Source: CAD feature listing. Evaluate the final solid. Frame: model axes, mm. Face numbers are marked on the shaded views. A direction names the side the tool comes from. Coordinates: 2 decimals unless noted, no trailing zeros. Loops run counter-clockwise (first coordinate to the right, second up) from the corner with the lowest first, then second, coordinate; pieces in that order, holes last. Notation, with made-up numbers: (53, -36) -> (61, -36) arc R35 cw to (61, 2) -> close; hole circle Ø1 at (15, 4). An arc over 180 degrees is marked (long way). Answer as CSV lines item,"result".
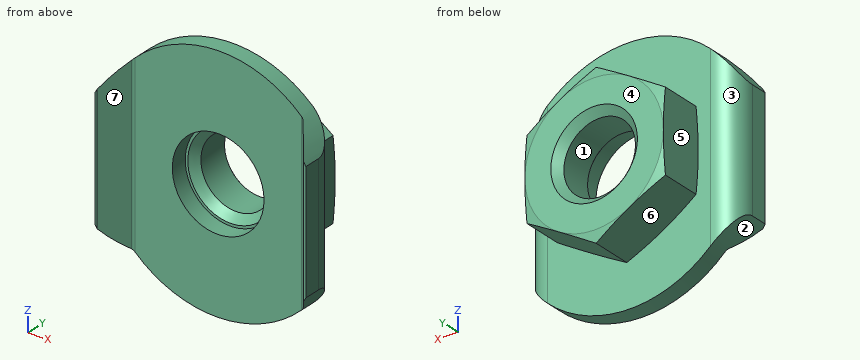
Autodesk Inventor part; units mm, degrees
ref_plane "FS1_XY" through (0, 0, 0) normal (0, 1, 0) x (1, 0, 0)
ref_plane "FS1_YZ" through (0, 0, 0) normal (1, 0, 0) x (0, 0, -1)
ref_plane "FS1_ZX" through (0, 0, 0) normal (0, 0, -1) x (0, 1, 0)
sketch "Skizze_1" plane through (0, 0, 0) normal (0, 0, 1) x (1, 0, 0)
  line L0 (-6.094, 2.6187) -> (-5.9701, 2.6187)
  line L1 (-5.9701, 2.6187) -> (-4.9601, 3.9225)
  arc A0 (-4.8019, 4) -> (-4.9601, 3.9225) centre (-4.8019, 3.8) ccw
  line L2 (-4.8019, 4) -> (4.8019, 4)
  arc A1 (4.9601, 3.9225) -> (4.8019, 4) centre (4.8019, 3.8) ccw
  line L3 (4.9601, 3.9225) -> (5.9701, 2.6187)
  line L4 (5.9701, 2.6187) -> (6.094, 2.6187)
  line L5 (6.094, 2.6187) -> (6.094, 3.606)
  arc A2 (6.094, 3.606) -> (4.7, 5) centre (4.7, 3.606) ccw
  line L6 (4.7, 5) -> (-4.7, 5)
  arc A3 (-4.7, 5) -> (-6.094, 3.606) centre (-4.7, 3.606) ccw
  line L7 (-6.094, 3.606) -> (-6.094, 2.6187)
extrude "Extrusion1" add sketch "Skizze_1" along normal mid plane 14
sketch "Skizze_2" plane through (0, 0, 0) normal (0, 0, 1) x (1, 0, 0)
  line L0 (0, 5) -> (0, 7.7)
  line L1 (0, 7.7) -> (4, 7.7)
  line L2 (4, 7.7) -> (4.8, 7.4856)
  line L3 (4.8, 7.4856) -> (4.8, 5.2144)
  line L4 (4.8, 5.2144) -> (4, 5)
  line L5 (4, 5) -> (0, 5)
  line L6 (0, 5) -> (0, 7.7)
revolve "Revolution1" add sketch "Skizze_2" angle 360 about axis through (0, 5, 0) along (0, -1, 0)
sketch "Skizze_3" plane through (0, 5, 0) normal (0, 1, 0) x (1, 0, 0)
  line L0 (-20, -18) -> (19, -18)
  line L1 (19, -18) -> (19, 12)
  line L2 (19, 12) -> (-20, 12)
  line L3 (-20, 12) -> (-20, -18)
  line L4 (-4, -2.3094) -> (0, -4.6188)
  line L5 (0, -4.6188) -> (4, -2.3094)
  line L6 (4, -2.3094) -> (4, 2.3094)
  line L7 (4, 2.3094) -> (0, 4.6188)
  line L8 (0, 4.6188) -> (-4, 2.3094)
  line L9 (-4, 2.3094) -> (-4, -2.3094)
extrude "Extrusion2" cut sketch "Skizze_3" along normal blind 2.7
sketch "Skizze_4" plane through (0, 0, 0) normal (0, 1, 0) x (-1, 0, 0)
  line L0 (23, 26) -> (-35, 26)
  line L1 (-35, 26) -> (-35, -16)
  line L2 (-35, -16) -> (23, -16)
  line L3 (23, -16) -> (23, 26)
  circle A0 centre (0, 0) radius 7
extrude "Extrusion3" cut sketch "Skizze_4" along normal blind 10
sketch "Skizze_5_ALT_Drilling_1" plane through (0, 0, 0) normal (0, 0, 1) x (1, 0, 0)
  line L0 (0, 4) -> (0, 7.7)
  line L1 (0, 7.7) -> (2.5, 7.7)
  line L2 (2.5, 7.7) -> (2.067, 7.267)
  line L3 (2.067, 7.267) -> (2.067, 5.433)
  line L4 (2.067, 5.433) -> (2.5, 5)
  line L5 (2.5, 5) -> (2.65, 5)
  line L6 (2.65, 5) -> (2.65, 4)
  line L7 (2.65, 4) -> (0, 4)
  line L8 (0, 4) -> (0, 7.7)
revolve "Revolution2" cut sketch "Skizze_5_ALT_Drilling_1" angle 360 about axis through (0, 4, 0) along (0, -1, 0)
thread "Thread1"
ref_plane "FS1_XY" through (0, 0, 0) normal (0, 1, 0) x (1, 0, 0)
ref_plane "FS1_YZ" through (0, 0, 0) normal (1, 0, 0) x (0, 0, -1)
ref_plane "FS1_ZX" through (0, 0, 0) normal (0, 0, -1) x (0, 1, 0)
ref_plane "FS2_XY" through (0, 0, 0) normal (0, 0, 1) x (1, 0, 0)
ref_plane "FS2_YZ" through (0, 0, 0) normal (1, 0, 0) x (0, 1, 0)
ref_plane "FS2_ZX" through (0, 0, 0) normal (0, 1, 0) x (0, 0, 1)
properties part number "102111-M-KOMP"
(1) Material intervals for L1, parallel to Z at x = 0, y = 4.4; L2, parallel to Y at x = 1.75, z = -3.75; L3, parallel to Y at x = -3.25, z = 1.75, sorted ascending. Write a range as [from, to].
Computed values:
L1,"[-7, -2.65], [2.65, 7]"
L2,"[4, 5]"
L3,"[4, 7.7]"
(2) Pin query (flat end, axial travel): pin 1 Ø4 at (x, z) = (-1.5, -1) entering from -Y; pin 2 Ø1 at (x, y) = (4.5, 4) entering from +Z; pin 3 Ø2 at (x, y) = (3, 7) entering from +Z. Return the tip coordinate at first contact, or that it passes through.
Computed values:
pin 1,"y = 4"
pin 2,"z = 5.74"
pin 3,"z = 3.46"
(3) Cut plane D-D (x = -4.5). Return the cut outline in (y, z), then the cut area to 3 significant figures.
Computed values:
outline,"(4, -5.36) -> (5, -5.36) -> (5, 5.36) -> (4, 5.36) -> close"
area,"10.7 mm^2"
(4) Cut plane C-C (z = -6). Return the cut outline in (x, y), then the cut area to 3 significant figures.
Computed values:
outline,"(-3.61, 4) -> (3.61, 4) -> (3.61, 5) -> (-3.61, 5) -> close"
area,"7.21 mm^2"
(5) Access query for the marked faces 4, 5, 6 and 7. Directions: +Z, -Z, +X, -X, +Y, -Y. A direction counts if a zero-diameter tool reaches every point of the face in a straight line with its end or side. Return the directions, or none.
Computed values:
face 4,"+Z, -Z, +X, -X, +Y"
face 5,"+Z, -Z, -X, +Y"
face 6,"-Z, -X, +Y"
face 7,"+Z, -Z, -Y"
(6) Cut plane A-A (y = 5.65). Return the cut outline in (x, z).
Computed values:
outline,"(-4, -2.31) -> (0, -4.62) -> (4, -2.31) -> (4, 2.31) -> (0, 4.62) -> (-4, 2.31) -> close; hole circle Ø4.13 at (0, 0)"
(7) Cut plane B-B (y = 3.1). Return the cut outline in (x, z).
Computed values:
outline,"(-6.09, -3.44) arc R7 ccw to (-5.6, -4.2) -> (-5.6, 4.2) arc R7 ccw to (-6.09, 3.44) -> close; (5.6, -4.2) arc R7 ccw to (6.09, -3.44) -> (6.09, 3.44) arc R7 ccw to (5.6, 4.2) -> close"
(8) Draft query along X for the marked faces 1, 2 and 3. Return one class per face: released by +X, released by -X, zero draft, split by the parting line, or undercut.
Computed values:
face 1,"undercut"
face 2,"split by the parting line"
face 3,"released by -X"
